Check sheet for the modelled part. Datum: model origin and axes. Units: mm. A direction names the side the tool comes from. Round coordinates to 2 decimals unless told otherwise and drop trailing zeros. Write each loop counter-clockwise with the first axis right and the second up, starting at its lowest first coordinate (ties: lowest second). Pieces come first, ordered by that corner, then holes. Notation, with made-up numbers: (5.25, -2) - (55.25, -2) arc R17 ccw to (55.25, 18) - close; hole circle Ø1 at (52, -27.5). An arc over 180 degrees is marked (long way). Answer as a JSON object with one key per item and string values. Group by question number.
Item 1: Gauge pin test, flat ends, axial feed: P1, Ø12, axis at y = 12, z = 5, coming from the +X side; P2, Ø2, axis at y = 7.5, z = 6, coming from the -X side; P3, Ø11.5, axis at x = -63.04, z = 7.94, coming from the +Y side; P4, Ø5, axis at x = -63.04, z = 7.94, coming from the -Y side. Record the tip position at first contact, or that the pin passes through.
Item 2: Sectioned sample at B-B on z = 6.5. Record the boundary of the cut face in (x, y).
Item 3: Release check for a two-part mould opening along Z. For faces 4 (the flat face through (13, -9.298, 16)), 5 (the flat face through (-25, 12, 31.75)), 6 (the flat face through (-62, -2.948, 27)) record: pulls with the +Z half, pulls with the -Z half, needs draft (parallel to the pull), parting line crosses it, or undercut.
Item 4: Sectioned sample at C-C on x = 12.5. Record the boundary of the cut face in (y, z), plus the area to 3 significant figures.
Item 5: Set-up check for faces 1 (the cylindrical face through (9.206, 4.119, 8.901)), 2 (the flat face through (-67.798, -3, 16)), 3 (the flat face through (-58.273, -6, 16)): record each of +Z, -Z, +X, -X, +Y, -Y from which the full face is reachable in a straight line by a thin tool's end or side.
Item 6: Sectioned sample at D-D on z = 15. Record the boundary of the cut face in (x, y), plus the area to 3 significant figures.
Item 7: Thickness scan on line 1 (Z direction, x = 13, y = 12); line 2 (X direction, y = 5.25, z = 20); line 3 (Z direction, x = 13, y = -6.25). Record the ranges inside material, lowest first.
Item 8: Sectioned sample at A-A on y = 1.75. Count the separate pieces of the cut face and the enclosed holes in it, plus the area to 3 significant figures.
```python
from build123d import *

# Parameters (mm, degrees)
BOSS_EXTRUDE1_DEPTH = 31.75
SKETCH2_R           = 3.175
CUT_EXTRUDE1_DEPTH  = 37.084
SKETCH3_R           = 4.445
CUT_EXTRUDE2_DEPTH  = 37.084


with BuildPart() as part:
    # Sketch1 → Boss-Extrude1 (new body)
    with BuildSketch(Plane.XY):
        with BuildLine():
            Line((-58.273322186, -9.297932879), (-58.273322186, -3.041379021))
            ThreePointArc((-58.273322186, -3.041379021), (-54.553578308, 5.9388771), (-45.573322186, 9.658620979))
            Line((-45.573322186, 9.658620979), (-3.917322186, 9.658620979))
            ThreePointArc((-3.917322186, 9.658620979), (5.062933935, 5.9388771), (8.782677814, -3.041379021))
            Line((8.782677814, -3.041379021), (8.782677814, -9.297932879))
            Line((8.782677814, -9.297932879), (18.307677814, -9.297932879))
            Line((18.307677814, -9.297932879), (18.307677814, 3.346975696))
            ThreePointArc((18.307677814, 3.346975696), (14.587933935, 12.327231817), (5.607677814, 16.046975696))
            Line((5.607677814, 16.046975696), (-55.098322186, 16.046975696))
            ThreePointArc((-55.098322186, 16.046975696), (-64.078578308, 12.327231817), (-67.798322186, 3.346975696))
            Line((-67.798322186, 3.346975696), (-67.798322186, -9.297932879))
            Line((-67.798322186, -9.297932879), (-58.273322186, -9.297932879))
        make_face()
    extrude(amount=BOSS_EXTRUDE1_DEPTH)

    # Sketch2 → Cut-Extrude1 (cut)
    with BuildSketch(Plane.XZ.offset(9.297932879)):
        with Locations(Location((-63.035822186, 7.9375, 0), (0, 0, 270))):
            Circle(SKETCH2_R)
        with Locations(Location((-63.035822186, 23.8125, 0), (0, 0, 270))):
            Circle(SKETCH2_R)
        with Locations(Location((13.545177814, 23.8125, 0), (0, 0, 270))):
            Circle(SKETCH2_R)
        with Locations(Location((13.545177814, 7.9375, 0), (0, 0, 270))):
            Circle(SKETCH2_R)
    extrude(amount=-CUT_EXTRUDE1_DEPTH, mode=Mode.SUBTRACT)

    # Sketch3 → Cut-Extrude2 (cut)
    with BuildSketch(Plane(origin=(0, -2.947932879, 0), x_dir=(-1, 0, 0), z_dir=(0, -1, 0))):
        with Locations(Location((-13.545177814, -23.8125, 0), (0, 0, 90))):
            Circle(SKETCH3_R)
        with Locations(Location((-13.545177814, -7.9375, 0), (0, 0, 90))):
            Circle(SKETCH3_R)
        with Locations(Location((63.035822186, -23.8125, 0), (0, 0, 90))):
            Circle(SKETCH3_R)
        with Locations(Location((63.035822186, -7.9375, 0), (0, 0, 90))):
            Circle(SKETCH3_R)
    extrude(amount=-CUT_EXTRUDE2_DEPTH, mode=Mode.SUBTRACT)


solid = part.part
```
Completed:
{
 "1": {"P1": "x = 18.03", "P2": "x = -67.4", "P3": "y = 15.86", "P4": "through"},
 "2": {"outline": "(-67.8, -9.3) - (-65.87, -9.3) - (-65.87, -2.95) - (-67.24, -2.95) - (-67.24, 7.06) arc R12.7 ccw to (-67.8, 3.35) - close; (-60.2, -9.3) - (-58.27, -9.3) - (-58.27, -3.04) arc R12.7 cw to (-45.57, 9.66) - (-3.92, 9.66) arc R12.7 cw to (8.78, -3.04) - (8.78, -9.3) - (10.71, -9.3) - (10.71, -2.95) - (9.34, -2.95) - (9.34, 15.49) arc R12.7 ccw to (5.61, 16.05) - (-55.1, 16.05) arc R12.7 ccw to (-58.83, 15.49) - (-58.83, -2.95) - (-60.2, -2.95) - close; (16.38, -9.3) - (18.31, -9.3) - (18.31, 3.35) arc R12.7 ccw to (17.75, 7.06) - (17.75, -2.95) - (16.38, -2.95) - close"},
 "3": {"face 4": "needs draft", "face 5": "pulls with the +Z half", "face 6": "undercut"},
 "4": {"outline": "(-9.3, 0) - (14.01, 0) - (14.01, 3.62) - (-2.95, 3.62) - (-2.95, 4.94) - (-9.3, 4.94) - close; (-9.3, 10.94) - (-2.95, 10.94) - (-2.95, 12.26) - (14.01, 12.26) - (14.01, 19.49) - (-2.95, 19.49) - (-2.95, 20.81) - (-9.3, 20.81) - close; (-9.3, 26.81) - (-2.95, 26.81) - (-2.95, 28.13) - (14.01, 28.13) - (14.01, 31.75) - (-9.3, 31.75) - close", "area": "371 mm²"},
 "5": {"face 1": "+Y", "face 2": "+Z, -Z, -X, +Y, -Y", "face 3": "+Z, -Z, -Y"},
 "6": {"outline": "(-67.8, -9.3) - (-58.27, -9.3) - (-58.27, -3.04) arc R12.7 cw to (-45.57, 9.66) - (-3.92, 9.66) arc R12.7 cw to (8.78, -3.04) - (8.78, -9.3) - (18.31, -9.3) - (18.31, 3.35) arc R12.7 ccw to (5.61, 16.05) - (-55.1, 16.05) arc R12.7 ccw to (-67.8, 3.35) - close", "area": "911 mm²"},
 "7": {"line 1": "0 to 3.53, 12.35 to 19.4, 28.22 to 31.75", "line 2": "-67.65 to -65.32, -60.75 to -55.19, 5.7 to 11.26, 15.83 to 18.16", "line 3": "0 to 4.81, 11.07 to 20.68, 26.94 to 31.75"},
 "8": {"separate pieces": "2", "enclosed holes": "4", "area": "416 mm²"}
}
